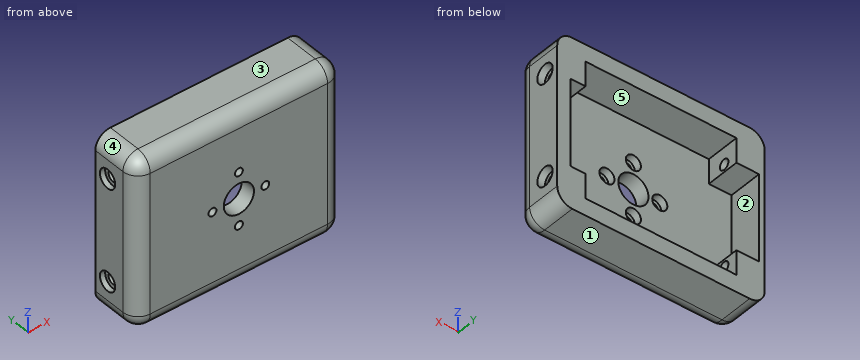
from build123d import *

# Parameters (mm, degrees)
SKETCH1_W           = 55
SKETCH1_H           = 45
BOSS_EXTRUDE1_DEPTH = 13
SKETCH2_W           = 40
SKETCH2_H           = 36
SKETCH2_W_2         = 6
SKETCH2_H_2         = 23
SKETCH2_W_3         = 4
CUT_EXTRUDE1_DEPTH  = 9
SKETCH3_R           = 1.4
CUT_EXTRUDE2_DEPTH  = 61.829680256
SKETCH4_R           = 1.05
SKETCH4_R_2         = 4
CUT_EXTRUDE3_DEPTH  = 37.653785616
SKETCH5_R           = 2
CUT_EXTRUDE4_DEPTH  = 2
SKETCH6_R           = 2.5
CUT_EXTRUDE5_DEPTH  = 1.4
CUT_EXTRUDE6_START  = -2
SKETCH7_R           = 2.5
CUT_EXTRUDE6_DEPTH  = 2
FILLET1_R           = 4


with BuildPart() as part:
    # Sketch1 → Boss-Extrude1 (new body)
    with BuildSketch(Plane(origin=(0, 0, 0), x_dir=(1, 0, 0), z_dir=(0, 1, 0))):
        Rectangle(SKETCH1_W, SKETCH1_H)
    extrude(amount=BOSS_EXTRUDE1_DEPTH)

    # Sketch2 → Cut-Extrude1 (cut)
    with BuildSketch(Plane(origin=(0, 13, 0), x_dir=(1, 0, 0), z_dir=(0, 1, 0))):
        Rectangle(SKETCH2_W, SKETCH2_H)
        with Locations((-23, 0)):
            Rectangle(SKETCH2_W_2, SKETCH2_H_2)
        with Locations((22, 0)):
            Rectangle(SKETCH2_W_3, SKETCH2_H_2)
    extrude(amount=-CUT_EXTRUDE1_DEPTH, mode=Mode.SUBTRACT)

    # Sketch3 → Cut-Extrude2 (cut, through all)
    with BuildSketch(Plane.ZY.offset(27.5)):
        with Locations((-13.5, 9)):
            Circle(SKETCH3_R)
        with Locations((13.5, 9)):
            Circle(SKETCH3_R)
    extrude(amount=-CUT_EXTRUDE2_DEPTH, mode=Mode.SUBTRACT)

    # Sketch4 → Cut-Extrude3 (cut, through all)
    with BuildSketch(Plane(origin=(0, 4, 0), x_dir=(1, 0, 0), z_dir=(0, 1, 0))):
        with Locations(Location((0, 7, 0), (0, 0, 270))):
            Circle(SKETCH4_R)
        with Locations(Location((7, 0, 0), (0, 0, 270))):
            Circle(SKETCH4_R)
        with Locations(Location((-7, 0, 0), (0, 0, 270))):
            Circle(SKETCH4_R)
        with Locations(Location((0, -7, 0), (0, 0, 270))):
            Circle(SKETCH4_R)
        with Locations(Location((0, 0, 0), (0, 0, 270))):
            Circle(SKETCH4_R_2)
    extrude(amount=-CUT_EXTRUDE3_DEPTH, mode=Mode.SUBTRACT)

    # Sketch5 → Cut-Extrude4 (cut)
    with BuildSketch(Plane(origin=(0, 4, 0), x_dir=(1, 0, 0), z_dir=(0, 1, 0))):
        with Locations(Location((-7, 0, 0), (0, 0, 270))):
            Circle(SKETCH5_R)
        with Locations(Location((0, 7, 0), (0, 0, 270))):
            Circle(SKETCH5_R)
        with Locations(Location((7, 0, 0), (0, 0, 270))):
            Circle(SKETCH5_R)
        with Locations(Location((0, -7, 0), (0, 0, 270))):
            Circle(SKETCH5_R)
    extrude(amount=-CUT_EXTRUDE4_DEPTH, mode=Mode.SUBTRACT)

    # Sketch6 → Cut-Extrude5 (cut)
    with BuildSketch(Plane.ZY.offset(27.5)):
        with Locations((-13.5, 9)):
            Circle(SKETCH6_R)
        with Locations((13.5, 9)):
            Circle(SKETCH6_R)
    extrude(amount=-CUT_EXTRUDE5_DEPTH, mode=Mode.SUBTRACT)

    # Sketch7 → Cut-Extrude6 (cut)
    with BuildSketch(Plane(origin=(27.5, 0, 0), x_dir=(0, 0, -1), z_dir=(1, 0, 0)).offset(CUT_EXTRUDE6_START)):
        with Locations(Location((-13.5, 9, 0), (0, 0, 180))):
            Circle(SKETCH7_R)
        with Locations(Location((13.5, 9, 0), (0, 0, 180))):
            Circle(SKETCH7_R)
    extrude(amount=CUT_EXTRUDE6_DEPTH, mode=Mode.SUBTRACT)

    # Fillet1
    fillet1_edges = [part.edges().sort_by_distance(p)[0] for p in [
        (0, 0, -22.5),
        (27.5, 0, 0),
        (0, 0, 22.5),
        (-27.5, 0, 0),
        (-27.5, 6.5, -22.5),
        (27.5, 6.5, -22.5),
        (27.5, 6.5, 22.5),
        (-27.5, 6.5, 22.5),
    ]]
    fillet(fillet1_edges, radius=FILLET1_R)


solid = part.part
Model file for the job. Use its own axes, mm. Face numbers are marked on the shaded views. A direction names the side the tool comes from. Coordinates: 2 decimals unless noted, no trailing zeros. Order: outer loops, then holes, each group sorted by start corner. A loop starts at its lowest first (then second) coordinate and runs counter-clockwise, first axis right, second up. Notation, with made-up numbers: M -16,24.25 L 29,24.25 A33 cw 29,61.25 Z; hole C 81.5,-4 d4. An arc over 180 degrees is marked long. Return JSON: item names as keys, results as strings.
1. Tool access for the marked faces 1 and 2: list every direction of +Z, -Z, +X, -X, +Y, -Y with a clear straight run to the whole face (end or side of a thin tool).
Ans:
{"face 1": "-Z, +X, -X, +Y, -Y", "face 2": "+Y"}
2. Saw through at A-A (x = -7). Give the cut face in (y, z), and give its area (3 significant figures).
Ans:
{"outline": "M 0,-18.5 A4 ccw 4,-22.5 L 13,-22.5 L 13,-18 L 4,-18 L 4,-2 L 2,-2 L 2,-1.05 L 0,-1.05 Z; M 0,1.05 L 2,1.05 L 2,2 L 4,2 L 4,18 L 13,18 L 13,22.5 L 4,22.5 A4 ccw 0,18.5 Z", "area": "242 mm^2"}
3. Flat gauge pins, fed straight in: pin 1 (5 mm diameter, centred on x = -10, z = -8.5, fed in from +Y); pin 2 (3 mm diameter, centred on y = 9, z = 13.5, fed in from -X). Where does each tip first touch, or does it go through?
Ans:
{"pin 1": "y = 4", "pin 2": "x = -26.1"}
4. Saw through at B-B (z = 0). Give the number of separate pieces and of enclosed holes in the cut face, and give its area (3 significant figures).
Ans:
{"separate pieces": "4", "enclosed holes": "0", "area": "202 mm^2"}
5. Pull direction X, two halves, no side cores. Call the marked faces 3, 4 and 5: +X half, -X half, draft (parallel to the pull), parting line (faces both ways), or undercut.
Ans:
{"face 3": "draft", "face 4": "-X half", "face 5": "undercut"}
6. Saw through at D-D (y = 5.5). Give the cut face in (x, z).
Ans:
{"outline": "M -27.5,-18.5 A4 ccw -23.5,-22.5 L 23.5,-22.5 A4 ccw 27.5,-18.5 L 27.5,18.5 A4 ccw 23.5,22.5 L -23.5,22.5 A4 ccw -27.5,18.5 Z; hole M -26,-11.5 L -20,-11.5 L -20,-18 L 20,-18 L 20,-11.5 L 24,-11.5 L 24,11.5 L 20,11.5 L 20,18 L -20,18 L -20,11.5 L -26,11.5 Z"}
7. Drill centre lines: probe 1 along Z at (x, y) = (-11.5, 9.5); probe 2 along X at (y, z) = (9.25, -1); probe 3 along Z at (x, y) = (22, 5.5). Where is each one in solid material? Low to high.
Ans:
{"probe 1": "-22.5 to -18, 18 to 22.5", "probe 2": "-27.5 to -26, 24 to 27.5", "probe 3": "-22.5 to -11.5, 11.5 to 22.5"}
8. Saw through at C-C (z = 7). Give the cut face in (x, y), and give its area (3 significant figures).
Ans:
{"outline": "M -27.5,4 A4 ccw -23.5,0 L -1.05,0 L -1.05,2 L -2,2 L -2,4 L -26,4 L -26,13 L -27.5,13 Z; M 1.05,0 L 23.5,0 A4 ccw 27.5,4 L 27.5,13 L 24,13 L 24,4 L 2,4 L 2,2 L 1.05,2 Z", "area": "246 mm^2"}
